Here's the drawing with two shaded views (mm, measured from the low corner). I have some questions. A direction names the side the tool comes from. Give positions to 0.01 mm unless a question says otherwise; leave off trailing zeros. Loops run counter-clockwise (first coordinate to the right, second up) from the corner with the lowest first, then second, coordinate; pieces in that order, holes last.
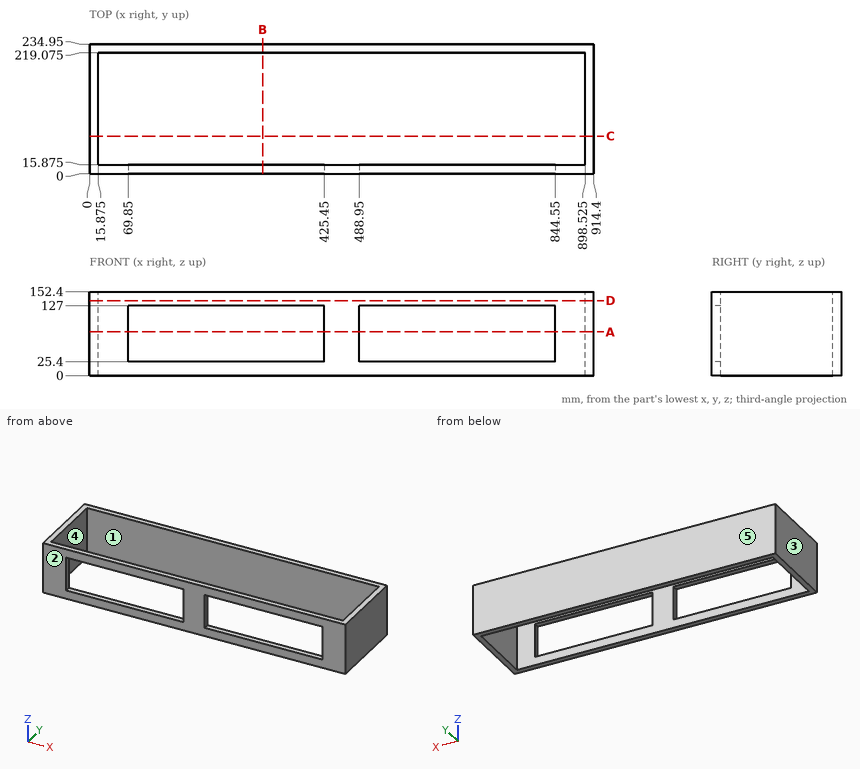
(1) Suppose I cut it at A-A on z = 79.5. List the corners of the cut face in (x, y) for me (3 decimals).
Returned:
outline: (0, 0) - (69.85, 0) - (69.85, 15.875) - (15.875, 15.875) - (15.875, 219.075) - (898.525, 219.075) - (898.525, 15.875) - (844.55, 15.875) - (844.55, 0) - (914.4, 0) - (914.4, 234.95) - (0, 234.95) - close; (425.45, 0) - (488.95, 0) - (488.95, 15.875) - (425.45, 15.875) - close
(2) Thinking about a two-plate mould opening in X: for the marked faces 3, 4 and 5, which applies, pulls with the +X half, pulls with the -X half, needs draft (parallel to the pull), parting line crosses it, or undercut?
Returned:
face 3: pulls with the -X half
face 4: undercut
face 5: needs draft
(3) Suppose I cut it at D-D on z = 136. List the corners of the cut face in (x, y) for me (3 decimals), plus the area to 3 significant figures.
Returned:
outline: (0, 0) - (914.4, 0) - (914.4, 234.95) - (0, 234.95) - close; hole (15.875, 15.875) - (898.525, 15.875) - (898.525, 219.075) - (15.875, 219.075) - close
area: 35,500 mm2
(4) Suppose I cut it at B-B on x = 314. List the corners of the cut face in (y, z) for me (3 decimals).
Returned:
outline: (0, 0) - (15.875, 0) - (15.875, 25.4) - (0, 25.4) - close; (0, 127) - (15.875, 127) - (15.875, 152.4) - (0, 152.4) - close; (219.075, 0) - (234.95, 0) - (234.95, 152.4) - (219.075, 152.4) - close
(5) Which directions (+Z, -Z, +X, -X, +Y, -Y) give clear straight access to the entire face, cutting with the end or side of a thin tool? Please do the marked faces 1 and 2.
Returned:
face 1: +Z, -Z
face 2: +Z, -Z, +X, -X, -Y
(6) Please list where these lines run through material, in increasing order: probe 1 along Y at (x, z) = (436, 26) (3 decimals); probe 2 along X at (y, z) = (48.5, 28) (3 decimals); probe 3 along Z at (x, y) = (132, 14).
Returned:
probe 1: y = 0 to 15.875, 219.075 to 234.95
probe 2: x = 0 to 15.875, 898.525 to 914.4
probe 3: z = 0 to 25.4, 127 to 152.4
(7) Will this pin go through, and if not, where does the flat tip stop? P1, Ø10, axis at x = 769.5, z = 54.5, coming from the -Y side (3 decimals).
Returned:
P1: stops at y = 219.075
(8) Suppose I cut it at C-C on y = 68. List the corners of the cut face in (x, z) for me (3 decimals), plus the area to 3 significant figures.
Returned:
outline: (0, 0) - (15.875, 0) - (15.875, 152.4) - (0, 152.4) - close; (898.525, 0) - (914.4, 0) - (914.4, 152.4) - (898.525, 152.4) - close
area: 4,840 mm2
